Geometry check sheet. Reference: the model listing, model coordinates, mm. Give positions to 0.01 mm unless a question says otherwise; leave off trailing zeros. Loops run counter-clockwise (first coordinate to the right, second up) from the corner with the lowest first, then second, coordinate; pieces in that order, holes last. Notation, with made-up numbers: (-5.75, 74) -> (15.25, 74) arc R14 cw to (15.25, 83) -> close; hole circle Ø11 at (21, -8.5). An arc over 180 degrees is marked (long way). Write each question's results on one line, items separated by ' | '. Start each with the question number.
1) Draft check along Y on faces 1 (the face through (-16.39, 26.39, 3.94)), 2 (the face through (25, 55, 4)), 3 (the face through (0, 1, 0)). Enter one of: pulls with the +Y half, pulls with the -Y half, needs draft (parallel to the pull), parting line crosses it, or undercut.
2) Sectioned sample at D-D on z = 2.5. Count the separate pieces of the cut face and the enclosed holes in it, then the cut area to 3 significant figures.
3) Sectioned sample at C-C on y = 25. Record the cut outline in (x, z).
4) Sectioned sample at A-A on x = 0. Record the cut outline in (y, z), then the cut area to 3 significant figures.
5) Sectioned sample at B-B on y = -45. Record the cut outline in (x, z), then the cut area to 3 significant figures.
6) Scan lines: line 1 (Y direction, x = 0, z = 2.75); line 2 (Y direction, x = -17.5, z = 2.75); line 3 (Y direction, x = -1, z = 1.5). Record each from-to range of solid material in increasing order. Write a range as from..to.
```python
from build123d import *

# Parameters (mm, degrees)
SKETCH1_W           = 60
SKETCH1_H           = 120
SKETCH1_R           = 3.25
SKETCH1_R_2         = 12
BOSS_EXTRUDE1_DEPTH = 8
M3_TAPPED_HOLE1_D   = 2.5
M4_TAPPED_HOLE1_D   = 3.3
CHAMFER1_SIZE       = 0.5
CHAMFER2_SIZE       = 10


with BuildPart() as part:
    # Sketch1 → Boss-Extrude1 (new body)
    with BuildSketch(Plane.XY):
        Rectangle(SKETCH1_W, SKETCH1_H)
        with Locations((-17.5, -15)):
            Circle(SKETCH1_R, mode=Mode.SUBTRACT)
        with Locations((-17.5, -45)):
            Circle(SKETCH1_R, mode=Mode.SUBTRACT)
        with Locations((17.5, -45)):
            Circle(SKETCH1_R, mode=Mode.SUBTRACT)
        with Locations((17.5, -15)):
            Circle(SKETCH1_R, mode=Mode.SUBTRACT)
        with Locations((0, 25)):
            Circle(SKETCH1_R_2, mode=Mode.SUBTRACT)
    extrude(amount=BOSS_EXTRUDE1_DEPTH)

    # M3 Tapped Hole1 (through all)
    with Locations(Plane.XY.offset(8)):
        with Locations((-13.788582233, 38.788582233), (-13.788582233, 11.211417767), (13.788582233, 11.211417767), (13.788582233, 38.788582233)):
            Hole(M3_TAPPED_HOLE1_D / 2)

    # M4 Tapped Hole1 (through all)
    with Locations(Plane.XY.offset(8)):
        with Locations((-15.5, 25), (0, 40.5), (15.5, 25), (0, 9.5)):
            Hole(M4_TAPPED_HOLE1_D / 2)

    # Chamfer1
    chamfer1_edges = [part.edges().sort_by_distance(p)[0] for p in [
        (-12, 25, 8),
    ]]
    chamfer(chamfer1_edges, length=CHAMFER1_SIZE)

    # Chamfer2
    chamfer2_edges = [part.edges().sort_by_distance(p)[0] for p in [
        (-30, 60, 4),
        (30, 60, 4),
    ]]
    chamfer(chamfer2_edges, length=CHAMFER2_SIZE)


solid = part.part
```
Result:
1) face 1: undercut | face 2: pulls with the +Y half | face 3: needs draft
2) separate pieces: 1 | enclosed holes: 13 | area: 6,460 mm^2
3) outline: (-30, 0) -> (-17.15, 0) -> (-17.15, 8) -> (-30, 8) -> close; (-13.85, 0) -> (-12, 0) -> (-12, 7.5) -> (-12.5, 8) -> (-13.85, 8) -> close; (12, 0) -> (13.85, 0) -> (13.85, 8) -> (12.5, 8) -> (12, 7.5) -> close; (17.15, 0) -> (30, 0) -> (30, 8) -> (17.15, 8) -> close
4) outline: (-60, 0) -> (7.85, 0) -> (7.85, 8) -> (-60, 8) -> close; (11.15, 0) -> (13, 0) -> (13, 7.5) -> (12.5, 8) -> (11.15, 8) -> close; (37, 0) -> (38.85, 0) -> (38.85, 8) -> (37.5, 8) -> (37, 7.5) -> close; (42.15, 0) -> (60, 0) -> (60, 8) -> (42.15, 8) -> close | area: 715 mm^2
5) outline: (-30, 0) -> (-20.75, 0) -> (-20.75, 8) -> (-30, 8) -> close; (-14.25, 0) -> (14.25, 0) -> (14.25, 8) -> (-14.25, 8) -> close; (20.75, 0) -> (30, 0) -> (30, 8) -> (20.75, 8) -> close | area: 376 mm^2
6) line 1: -60..7.85, 11.15..13, 37..38.85, 42.15..60 | line 2: -60..-48.25, -41.75..-18.25, -11.75..60 | line 3: -60..8.19, 10.81..13.04, 36.96..39.19, 41.81..60
